CAD build for the part. Positions are in the model's coordinates, mm. Face numbers are marked on the shaded views. A direction names the side the tool comes from. Coordinates: 2 decimals unless noted, no trailing zeros. Loops run counter-clockwise (first coordinate to the right, second up) from the corner with the lowest first, then second, coordinate; pieces in that order, holes last. Notation, with made-up numbers: M 57,18 L 86,18 A30 ccw 86,54 Z; hole C 75,-20 d2. An arc over 180 degrees is marked long. Answer as a JSON object with one key per item and string values. Group by question number.
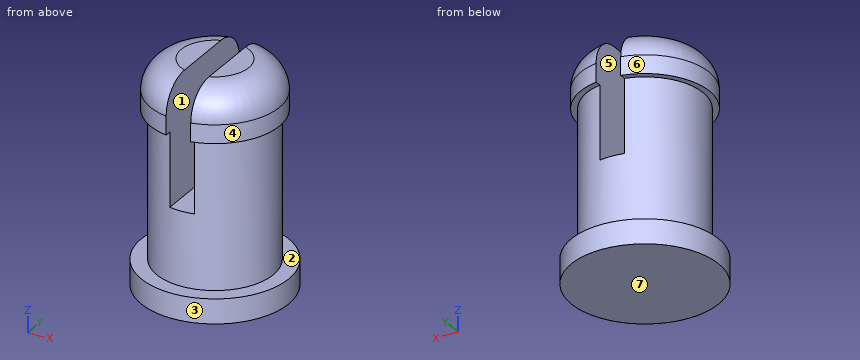
Autodesk Fusion 360 part; units mm, degrees
sketch "Boceto1" plane through (0, 0, 0) normal (0, 0, 1) x (1, 0, 0)
  circle A0 centre (0, 0) radius 6
  dimension "d1" = 12
extrude "Extruir1" add sketch "Boceto1" along normal blind 18
ref_plane "PlanoDeObra1" through (0, 0, 2) normal (0, 0, -1) x (-1, 0, 0)
sketch "Boceto2" plane through (0, 0, 2) normal (0, 0, -1) x (-1, 0, 0)
  circle A0 centre (0, 0) radius 4.75
  circle A1 centre (0, 0) radius 6
  dimension "d5" = 9.5
  dimension "d6" = 12
extrude "Extruir2" cut sketch "Boceto2" against normal blind 12
sketch "Boceto3" plane through (0, 0, 18) normal (0, 0, 1) x (-1, 0, 0)
  line L0 (-1, 7) -> (1, 7)
  line L1 (1, 7) -> (1, -7)
  line L2 (1, -7) -> (-1, -7)
  line L3 (-1, -7) -> (-1, 7)
  circle A0 centre (0, 0) radius 10
  circle A1 centre (0, 0) radius 6
  circle A2 centre (0, 0) radius 5.25
  circle A3 centre (0, 0) radius 6
  dimension "d11" = 2
  dimension "d12" = 1
  dimension "d15" = 10.5
  dimension "d16" = 12
extrude "Extruir3" cut sketch "Boceto3" against normal blind 10 contours L0 L1 L3 A1 A3 | L1 L3 A1 A2 A3 | L3 A1 A2 A3 | L1 A1 A2 A3 | L1 L3 A2 | L1 L2 L3 A1 A3 | L1 L3 A1 A2 A3
fillet "Empalme3" radius 2.5 2 edges at (5.25, 0, 18) (-5.25, 0, 18)
Item 1: Pull direction X, two halves, no side cores. Call the marked faces 5, 6 and 7: released by +X, released by -X, zero draft, split by the parting line, or undercut.
Item 2: Tool access for the marked faces 1, 2, 3 and 4: list every direction of +Z, -Z, +X, -X, +Y, -Y with a clear straight run to the whole face (end or side of a thin tool).
Item 3: Pin check, flat tips, straight feed: pin 1 (1.5 mm diameter, centred on x = 2, z = 13.5, fed in from +Y); pin 2 (6 mm diameter, centred on x = -2.5, z = 13.5, fed in from +Y); pin 3 (3 mm diameter, centred on y = -2.5, z = 14, fed in from -X). Stop position of each tip, or through.
Item 4: Slice it at C-C, the plane z = 7.5. Write the cut outline in (x, y), then the cut area to 3 significant figures.
Item 5: Slice it at B-B, the plane x = 0. Write the cut outline in (y, z).
Item 6: Drill centre lines: L1, parallel to Z at x = 5.25, y = -0.75; L2, parallel to X at y = 3, z = 11.5; L3, parallel to X at y = 2.25, z = 9.75. Where is each one in solid material? Low to high. Write a range as from..to.
Item 7: Slice it at A-A, the plane y = 0. Write the cut outline in (x, z), then the cut area to 3 significant figures.
Item 8: Slice it at D-D, the plane z = 10. Write the cut outline in (x, y), then the cut area to 3 significant figures.
Computed:
{
 "1": {"face 5": "undercut", "face 6": "released by -X", "face 7": "zero draft"},
 "2": {"face 1": "+Z, +Y, -Y", "face 2": "none", "face 3": "+Z, -Z", "face 4": "+Z, +X"},
 "3": {"pin 1": "y = 5.05", "pin 2": "y = 5.15", "pin 3": "x = -5.15"},
 "4": {"outline": "C 0,0 d9.5", "area": "70.9 mm2"},
 "5": {"outline": "M -6,0 L 6,0 L 6,2 L 4.75,2 L 4.75,8 L -4.75,8 L -4.75,2 L -6,2 Z"},
 "6": {"L1": "0..2", "L2": "-3.68..-1, 1..3.68", "L3": "-4.18..-1, 1..4.18"},
 "7": {"outline": "M -6,0 L 6,0 L 6,2 L 4.75,2 L 4.75,14 L 5.25,14 L 5.25,15.5 A2.5 ccw 2.75,18 L 1,18 L 1,8 L -1,8 L -1,18 L -2.75,18 A2.5 ccw -5.25,15.5 L -5.25,14 L -4.75,14 L -4.75,2 L -6,2 Z", "area": "157 mm2"},
 "8": {"outline": "M -1,-4.64 L -1,4.64 A4.75 ccw Z; M 1,-4.64 A4.75 ccw 1,4.64 Z", "area": "52.0 mm2"}
}
